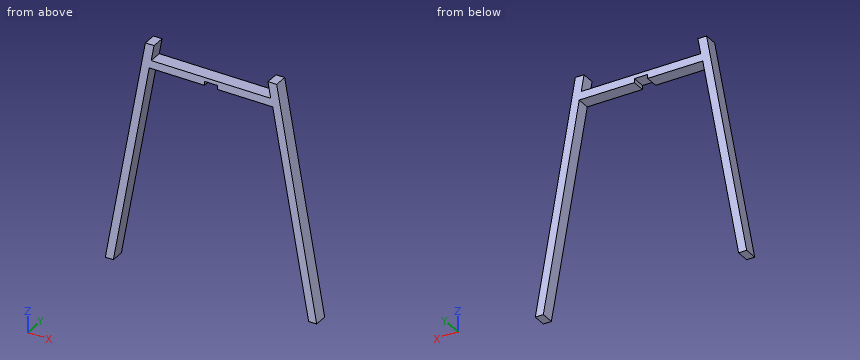
from build123d import *

# Parameters (mm, degrees)
F1_DEPTH = 12.5
F2_W     = 25
F2_H     = 7.5
F3_DEPTH = 12.5


with BuildPart() as f1:
    # F0 (on Front) → F1 (new body, symmetric)
    with BuildSketch(Plane.XZ):
        Polygon((-116.882713, 385), (0, 385), (0, 400), (-113.113844, 400), (-107.824034, 430), (-124.179398, 430), (-200, 0), (-184.768601, 0), align=None)
        Polygon((0, 400), (0, 385), (116.882713, 385), (184.768601, 0), (200, 0), (124.179398, 430), (107.824034, 430), (113.113844, 400), align=None)
    extrude(amount=F1_DEPTH, both=True)

    # F2 (on Front) → F3 (cut, symmetric)
    with BuildSketch(Plane.XZ):
        with Locations((0, 388.75)):
            Rectangle(F2_W, F2_H)
    extrude(amount=F3_DEPTH, both=True, mode=Mode.SUBTRACT)


solid = f1.part
The model under review builds one solid part; all positions refer to its coordinate system, in mm. Coordinates: 2 decimals unless noted, no trailing zeros. Loops run counter-clockwise (first coordinate to the right, second up) from the corner with the lowest first, then second, coordinate; pieces in that order, holes last.
(1) Wall thickness on L1, parallel to Z at x = -23.5, y = -0.25; L2, parallel to X at y = 5.75, z = 240; L3, parallel to X at y = 9.5, z = 143: over which ranges is each line inside the solid? List them lowest first.
Determined:
L1: z = 385 to 400
L2: x = -157.68 to -142.45, 142.45 to 157.68
L3: x = -174.79 to -159.55, 159.55 to 174.79
(2) Consider section B-B, the plane z = 104. Give the boundary of the cut face in (x, y), plus the area to 3 significant figures.
Determined:
outline: (-181.66, -12.5) - (-166.43, -12.5) - (-166.43, 12.5) - (-181.66, 12.5) - close; (166.43, -12.5) - (181.66, -12.5) - (181.66, 12.5) - (166.43, 12.5) - close
area: 762 mm2
(3) Consider section A-A, the plane y = 0.25. Give the boundary of the cut face in (x, z), plus the area to 3 significant figures.
Determined:
outline: (-200, 0) - (-184.77, 0) - (-116.88, 385) - (-12.5, 385) - (-12.5, 392.5) - (12.5, 392.5) - (12.5, 385) - (116.88, 385) - (184.77, 0) - (200, 0) - (124.18, 430) - (107.82, 430) - (113.11, 400) - (-113.11, 400) - (-107.82, 430) - (-124.18, 430) - close
area: 16,400 mm2
(4) Consider section C-C, the plane x = 87. Give the boundary of the cut face in (y, z).
Determined:
outline: (-12.5, 385) - (12.5, 385) - (12.5, 400) - (-12.5, 400) - close
(5) Consider section D-D, the plane x = -168. Give the boundary of the cut face in (y, z).
Determined:
outline: (-12.5, 95.1) - (12.5, 95.1) - (12.5, 181.48) - (-12.5, 181.48) - close
(6) Insertion check: P1, Ø10, axis at x = 84, y = -8, coming from the -Z side; P2, Ø7.5, axis at x = -5, y = -3.5, coming from the +Z side; P3, Ø1, axis at y = 9, z = 49, coming from the -X side. Each pin has a flat end and moves straight along its axis. Give the tip position at first contact, or say it passes through.
Determined:
P1: stops at z = 385
P2: stops at z = 400
P3: stops at x = -191.45
